```python
from build123d import *

# Parameters (mm, degrees)
F0_R      = 20.2439763863
F1_DEPTH  = 10.16
F2_R      = 12.3390116376
F3_DEPTH  = 8.89
F5_DEPTH  = 0.254
F6_DEPTH  = 0.254
F7_DEPTH  = 2.286
F8_DEPTH  = 2.286
F10_DEPTH = 25.4
F11_DEPTH = 50.8
F12_DEPTH = 1.27
F13_DEPTH = 1.27
F14_DEPTH = 25.4
F15_R     = 5.9555192151
F16_DEPTH = 167.64
F17_SIZE2 = 2.794
F17_SIZE  = 160.0681527963
F18_W     = 45.1150629669
F18_H     = 21.0420321673
F19_DEPTH = 25.4
F20_DEPTH = 25.4


with BuildPart() as f1:
    # F0 (on Top) → F1 (new body)
    with BuildSketch(Plane.XY):
        Circle(F0_R)
    extrude(amount=F1_DEPTH)

    # F2 (on face) → F3 (join)
    with BuildSketch(Plane.XY.offset(10.16)):
        Circle(F2_R)
    extrude(amount=F3_DEPTH)

    # F4 (on Front) → F5 (join)
    with BuildSketch(Plane.XZ):
        with BuildLine():
            add(Edge.make_bspline(
                [(-12.1147008613, 18.9316812903), (-12.5825885387, 39.643614737), (-14.1043760911, 180.4872847527), (-20.1423116849, 215.1594423433), (-16.5980636671, 214.2285434237), (-12.8136342596, 217.1071550637), (-13.8994905387, 225.3991797656), (-17.690195851, 229.7737918888), (-21.3235962144, 228.5443351063), (-21.72468447, 231.1706865689), (-23.0745608098, 250.4649690024), (-22.9518555989, 256.8313726894), (-25.9612755155, 279.5145026457), (-19.7421258922, 272.3476049684), (-8.8885956952, 268.998501799), (6.6271937698, 261.4946225406), (12.2027765589, 256.1934321206), (17.5689411606, 248.9539384021), (19.5820695948, 242.6412768865), (21.7285943019, 235.2163703421), (21.0795757322, 226.6989574981), (17.1180518063, 124.7114584437), (15.2094878956, 77.70771609), (11.6083548837, 18.1667354361), (12.5199184163, 13.1739974773), (7.8980496645, 11.3722942506), (0.3726356815, 13.3748423837), (-11.8699226938, 12.3427906017), (-12.0266797417, 15.035259866), (-12.1147008613, 18.9316812903)],
                knots=[0, 0, 0, 0, 0.1257254435, 0.1801466998, 0.1919036578, 0.2112403794, 0.2389108592, 0.261334308, 0.2775826335, 0.2907551098, 0.3325149493, 0.3636705446, 0.4039783899, 0.4240659342, 0.4586729556, 0.4992031799, 0.5266476396, 0.5552636706, 0.5809163826, 0.6063516787, 0.6344015668, 0.7303572224, 0.8074506533, 0.8789177389, 0.897509656, 0.9162026247, 0.9446563322, 0.976347968, 1, 1, 1, 1], degree=3))
        make_face()
    extrude(amount=F5_DEPTH)

    # F6 (add): a face of the model
    f6_faces = [f1.faces().sort_by_distance(p)[0] for p in [
        (0.2349858377, 0, 153.5959306446),
    ]]
    extrude(f6_faces, amount=F6_DEPTH)

    # F7 (add): a face of the model
    f7_faces = [f1.faces().sort_by_distance(p)[0] for p in [
        (0.2349858377, 0.254, 153.5959306446),
    ]]
    extrude(f7_faces, amount=F7_DEPTH)

    # F8 (add): a face of the model
    f8_faces = [f1.faces().sort_by_distance(p)[0] for p in [
        (0.2349858377, -0.254, 153.5959306446),
    ]]
    extrude(f8_faces, amount=F8_DEPTH)

    # F9 (on Front) → F10 (join)
    with BuildSketch(Plane.XZ):
        Polygon((-28.4392070025, 277.075022459), (5.8726719581, 261.9545459747), (-7.6194559224, 282.5416624546), align=None)
    extrude(amount=F10_DEPTH)

    # F11 (cut): a face of the model
    f11_faces = [f1.faces().sort_by_distance(p)[0] for p in [
        (-10.061996989, -25.4, 273.8570769628),
    ]]
    extrude(f11_faces, amount=-F11_DEPTH, mode=Mode.SUBTRACT)

    # F12 (cut): a face of the model
    f12_faces = [f1.faces().sort_by_distance(p)[0] for p in [
        (0.248434517, -2.54, 153.5481680876),
    ]]
    extrude(f12_faces, amount=-F12_DEPTH, mode=Mode.SUBTRACT)

    # F13 (cut): a face of the model
    f13_faces = [f1.faces().sort_by_distance(p)[0] for p in [
        (0.248434517, 2.54, 153.5481680876),
    ]]
    extrude(f13_faces, amount=-F13_DEPTH, mode=Mode.SUBTRACT)

    # F14 (cut): a face of the model
    f14_faces = [f1.faces().sort_by_distance(p)[0] for p in [
        (0.248434517, -1.27, 153.5481680876),
    ]]
    extrude(f14_faces, amount=-F14_DEPTH, mode=Mode.SUBTRACT)

    # F15 (on face) → F16 (join)
    with BuildSketch(Plane(origin=(0, 0, 0), x_dir=(1, 0, 0), z_dir=(0, 0, -1))):
        Circle(F15_R)
    extrude(amount=F16_DEPTH)

    # F17
    f17_edges = [f1.edges().sort_by_distance(p)[0] for p in [
        (-5.955519, 0, -167.64),
    ]]
    f17_side = f1.faces().sort_by_distance((-5.955519, 0, -83.82))[0]
    chamfer(f17_edges, length=F17_SIZE, length2=F17_SIZE2, reference=f17_side)

    # F18 (on Front) → F19 (cut)
    with BuildSketch(Plane.XZ):
        with Locations((1.2053744867, 10.5210160837)):
            Rectangle(F18_W, F18_H)
    extrude(amount=-F19_DEPTH, mode=Mode.SUBTRACT)

    # F20 (cut): a face of the model
    f20_faces = [f1.faces().sort_by_distance(p)[0] for p in [
        (0, 0, 8.3930130148),
    ]]
    extrude(f20_faces, amount=-F20_DEPTH, mode=Mode.SUBTRACT)


solid = f1.part
```
Geometry: final body of the model. Coordinates: model frame, mm. A direction names the side the tool comes from. Give positions to 0.01 mm unless a question says otherwise; leave off trailing zeros. Loops run counter-clockwise (first coordinate to the right, second up) from the corner with the lowest first, then second, coordinate; pieces in that order, holes last. Notation, with made-up numbers: (14.25, 3) - (63.25, 3) arc R22 ccw to (63.25, 24) - close; hole circle Ø5 at (-38.5, 32). An arc over 180 degrees is marked (long way). Answer as CSV lines item,"result". Start each with the question number.
(1) Reachability of faces 1 (the face through (0, 0, -167.64)), 2 (the face through (-4.535, -0.2, -88.726)) from +Z, -Z, +X, -X, +Y, -Y: full face, straight path, thin tool, end or side. Return the list, or none.
(2) Section query B-B (z = -10.5). Output: boundary loops of the cut face in (x, y), and give its area (3 significant figures).
(3) Section query A-A (z = -72). Output: boundary loops of the cut face in (x, y).
(4) Pin query (flat end, axial travel): P1, Ø4, axis at x = -2.5, z = -65.5, coming from the +Y side; P2, Ø4, axis at x = 4, z = -67.5, coming from the -Y side; P3, Ø1.5, axis at y = 1, z = -109, coming from the +X side. Return the tip coordinate at first contact, or that it passes through.
(5) Ray query, line 1 along Y through (x, z) = (-4, -57.5); line 2 along Y through (x, z) = (-0.25, -111.5); line 3 along X through (y, z) = (3, -95.5). Return the intervals inside material, ascending. Write a range as [from, to].
Worked answers:
1,face 1,"-Z, +X, -X, +Y, -Y"
1,face 2,"-Z"
2,outline,"circle Ø11.81 at (0, 0)"
2,area,"110 mm^2"
3,outline,"circle Ø9.66 at (0, 0)"
4,P1,"stops at y = 4.92"
4,P2,"stops at y = -4.48"
4,P3,"stops at x = 4.18"
5,line 1,"y = [-3.14, 3.14]"
5,line 2,"y = [-4.13, 4.13]"
5,line 3,"x = [-3.25, 3.25]"
